Input: part model. Units: mm. Frame: model coordinates. Face numbers are marked on the shaded views. A direction names the side the tool comes from. Give positions to 0.01 mm unless a question says otherwise; leave off trailing zeros. Write each loop counter-clockwise with the first axis right and the second up, starting at its lowest first coordinate (ties: lowest second). Pieces come first, ordered by that corner, then holes. Notation, with made-up numbers: (-13, 70.5) - (35, 70.5) arc R21 ccw to (35, 102.5) - close; hole circle Ø10 at (-2, 74). An arc over 180 degrees is marked (long way). Answer as CSV lines item,"result".
```python
from build123d import *

# Parameters (mm, degrees)
SKETCH1_R               = 5
BOSS_EXTRUDE1_DEPTH     = 20.355
CUT_EXTRUDE1_DEPTH      = 22.548225565
CIRPATTERN1_COUNT       = 8
CUT_EXTRUDE2_DEPTH      = 22.421117005
CUT_EXTRUDE2_DEPTH_BACK = 22.421117005
SKETCH4_R               = 1.6


with BuildPart() as part:
    # Sketch1 → Boss-Extrude1 (new body)
    with BuildSketch(Plane.XY):
        Circle(SKETCH1_R)
    extrude(amount=BOSS_EXTRUDE1_DEPTH)

    # Sketch2 → Cut-Extrude1 (cut, through all)
    with BuildSketch(Plane.XY):
        Polygon((0, 3.015315818), (-0.43705364, 3.420638152), (-1.367879142, 4.521896493), (-1.652539145, 4.719016251), (-1.899055149, 5.271190713), (0, 6.265180055), (1.899055149, 5.271190713), (1.652539145, 4.719016251), (1.367879142, 4.521896493), (0.43705364, 3.420638152), align=None)
    cut_extrude1 = extrude(amount=CUT_EXTRUDE1_DEPTH, mode=Mode.SUBTRACT)

    # CirPattern1: Cut-Extrude1 ×8 about axis
    cirpattern1_axis = Axis((0, 0, 0), (0, 0, 1))
    for i in range(1, CIRPATTERN1_COUNT):
        add(cut_extrude1.rotate(cirpattern1_axis, i * 360 / CIRPATTERN1_COUNT), mode=Mode.SUBTRACT)

    # Sketch4 → Cut-Extrude2 (cut, two sides: drawn at the far end of the back side and taken through both)
    with BuildSketch(Plane.XY.offset(20.355).offset(-CUT_EXTRUDE2_DEPTH_BACK)):
        Circle(SKETCH4_R)
    extrude(amount=CUT_EXTRUDE2_DEPTH + CUT_EXTRUDE2_DEPTH_BACK, mode=Mode.SUBTRACT)


solid = part.part
```
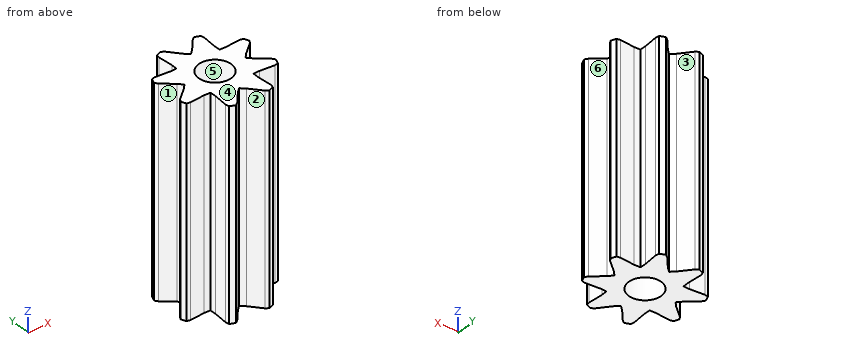
Item 1: Cut plane A-A on x = 1. Return the cut outline in (y, z) (3 decimals).
The answers:
outline,"(-4.087, 0) - (-1.249, 0) - (-1.249, 20.355) - (-4.087, 20.355) - close; (1.249, 0) - (4.087, 0) - (4.087, 20.355) - (1.249, 20.355) - close"
Item 2: Cut plane B-B on y = -0.75. Return the cut outline in (x, z) (3 decimals), plus the area to 3 significant figures.
The answers:
outline,"(-3.791, 0) - (-1.413, 0) - (-1.413, 20.355) - (-3.791, 20.355) - close; (1.413, 0) - (3.791, 0) - (3.791, 20.355) - (1.413, 20.355) - close"
area,"96.8 mm²"
Item 3: Ray query, line 1 (X direction, y = 4, z = 15.75); line 2 (Y direction, x = 1.25, z = 10); line 3 (X direction, y = 4.25, z = 14.25). Return the intervals inside material, ascending. Write a range as from..to.
The answers:
line 1,"-2.22..-0.93, 0.93..2.22"
line 2,"-4.38..-1, 1..4.38"
line 3,"-2.21..-1.14, 1.14..2.21"
Item 4: Contact query for a flat-ended pin moving along its axis: pin 1 (1.5 mm diameter, centred on x = -3.5, z = 17, fed in from -Y). Output: stop coordinate, or through.
The answers:
pin 1,"y = -2.23"
Item 5: Mould query, pull axis X, two halves, no side actions, for the marked faces 1, 2, 3 and 4. Classes: +X half, -X half, draft (parallel to the pull), parting line (faces both ways), or undercut.
The answers:
face 1,"-X half"
face 2,"undercut"
face 3,"undercut"
face 4,"draft"
Item 6: Cut plane C-C on x = -2.5. Return the cut outline in (y, z) (3 decimals).
The answers:
outline,"(-2.118, 0) - (2.118, 0) - (2.118, 20.355) - (-2.118, 20.355) - close"
Item 7: Reachability of the marked faces 5 and 6 from +Z, -Z, +X, -X, +Y, -Y: full face, straight path, thin tool, end or side. Return the list, or none.
The answers:
face 5,"+Z, -Z"
face 6,"+Z, -Z, +X"
